Part model, mm, in its own coordinate system. A direction names the side the tool comes from. Coordinates: 2 decimals unless noted, no trailing zeros. Loops run counter-clockwise (first coordinate to the right, second up) from the corner with the lowest first, then second, coordinate; pieces in that order, holes last. Notation, with made-up numbers: (77, 5.25) - (100, 5.25) arc R17 cw to (100, 13.25) - close; hole circle Ø10 at (89, 60.25). An arc over 180 degrees is marked (long way). Use a Markdown table: item, result. Add a question column.
1. Drop flat-ended pins along their axis: pin 1 (2 mm diameter, centred on x = 1, z = 5.5, fed in from -Y); pin 2 (0.5 mm diameter, centred on y = 1, z = 0, fed in from +X); pin 3 (2 mm diameter, centred on x = 1, z = 7, fed in from +Y). Give the stop position or say it passes through.
2. Band-saw the part on A-A, the plane z = 5. Give the cut face in (x, y), plus the area to 3 significant figures.
3. Pull direction Y, two halves, no side cores. Call faces 3 (the flat face through (0.7, 0.6, 0)), 4 (the conical face through (0.35, -0.05, 1.22)), 5 (the cylindrical face through (-2.23, -0.29, 1.35)): pulls with the +Y half, pulls with the -Y half, needs draft (parallel to the pull), parting line crosses it, or undercut.
4. 3-axis set-ups, long thin cutter, end or side, ignore diameter. For faces 1 (the cylindrical face through (-1.29, -0.17, 11.84)), 2 (the flat face through (-0.7, 0.6, 0)): which of +Z, -Z, +X, -X, +Y, -Y reach the whole face in a straight line?
5. Wall check: probe 1 along X at (y, z) = (-0.05, 6.75); probe 2 along Z at (x, y) = (-1.1, -1.15); probe 3 along X at (y, z) = (-0.45, 13.75). Give the ranges that are in metal, low to high. Write a range as [from, to].
Autodesk Inventor part; units mm, degrees
ref_plane "YZ Plane" through (0, 0, 0) normal (1, 0, 0) x (0, 1, 0)
ref_plane "XZ Plane" through (0, 0, 0) normal (0, 1, 0) x (-1, 0, 0)
ref_plane "XY Plane" through (0, 0, 0) normal (0, 0, 1) x (1, 0, 0)
sketch "スケッチ1" plane through (0, 0, 0) normal (1, 0, 0) x (0, 1, 0)
  line L0 (0, 21.7) -> (0, 0)
  line L1 (0, 0) -> (1.25, 0)
  line L2 (2.25, 1) -> (2.25, 1.7)
  line L3 (2.25, 1.7) -> (1.3, 1.7)
  line L4 (1.3, 1.7) -> (1.3, 21.7)
  line L5 (1.3, 21.7) -> (0, 21.7)
  line L6 (1.25, 0) -> (0, 1.7)
  arc A0 (1.25, 0) -> (2.25, 1) centre (1.25, 1) ccw
  line L7 (1.25, 0) -> (2.25, 0)
  line L8 (2.25, 0) -> (2.25, 1)
  dimension "d2" = 1.7
  dimension "d10" = 20
  dimension "d11" = 2.6
  dimension "d12" = 4.5
  dimension "d14" = 1
revolve "回転1" add sketch "スケッチ1" angle 360 about axis through (0, 0, 21.7) along (0, 0, -1) contours L5 L4 L3 L2 A0 L6 L0
thread "ねじ1"
sketch "スケッチ2" plane through (0, 0, 1.7) normal (0, 0, 1) x (1, 0, 0)
  line L0 (0.3339, -1.6357) -> (-0.3339, -1.6357)
  line L1 (-0.3339, -1.6357) -> (-0.3339, -0.7226)
  line L2 (-0.3339, 1.6357) -> (0.3339, 1.6357)
  line L3 (0.3339, 1.6357) -> (0.3339, 0.7226)
  line L4 (0.3339, -1.6357) -> (-0.3339, 1.6357) construction
  line L5 (-0.3339, -1.6357) -> (0.3339, 1.6357) construction
  line L6 (-1.5922, 0.2226) -> (-0.8339, 0.2226)
  line L7 (1.5922, 0.2226) -> (1.5922, -0.2226)
  line L8 (1.5922, -0.2226) -> (0.8339, -0.2226)
  line L9 (-1.5922, -0.2226) -> (-1.5922, 0.2226)
  line L10 (-1.5922, 0.2226) -> (1.5922, -0.2226) construction
  line L11 (1.5922, 0.2226) -> (-1.5922, -0.2226) construction
  circle A0 centre (0, 0) radius 2.25
  line L12 (0.3339, -0.7226) -> (0.3339, -1.6357)
  line L13 (0.8339, 0.2226) -> (1.5922, 0.2226)
  line L14 (-0.8339, -0.2226) -> (-1.5922, -0.2226)
  line L15 (-0.3339, 0.7226) -> (-0.3339, 1.6357)
  arc A1 (0.8339, -0.2226) -> (0.3339, -0.7226) centre (0.8339, -0.7226) ccw
  arc A2 (0.3339, 0.7226) -> (0.8339, 0.2226) centre (0.8339, 0.7226) ccw
  arc A3 (-0.8339, 0.2226) -> (-0.3339, 0.7226) centre (-0.8339, 0.7226) ccw
  arc A4 (-0.3339, -0.7226) -> (-0.8339, -0.2226) centre (-0.8339, -0.7226) ccw
  point P0 (0, 0)
  point P1 (-0.3339, -0.2226)
  point P2 (-0.3339, 0.2226)
  point P3 (0.3339, 0.2226)
  point P4 (0.3339, -0.2226)
  dimension "d18" = 0.5
extrude "押し出し2" add sketch "スケッチ2" against normal blind 1.7
revolve "回転2" cut sketch "スケッチ1" angle 360 about axis through (0, 0, 21.7) along (0, 0, -1) contours A0 L8 L7
properties part number "F-2620EB" material "チタン"
Geometry check:
| question | item | result |
|---|---|---|
| 1 | pin 1 | stops at y = -1.3 |
| 1 | pin 2 | stops at x = 1.66 |
| 1 | pin 3 | stops at y = 1.3 |
| 2 | outline | circle Ø2.6 at (0, 0) |
| 2 | area | 5.31 mm^2 |
| 3 | face 3 | needs draft |
| 3 | face 4 | undercut |
| 3 | face 5 | parting line crosses it |
| 4 | face 1 | +Z |
| 4 | face 2 | -Z, +X, -X, +Y, -Y |
| 5 | probe 1 | x = [-1.3, 1.3] |
| 5 | probe 2 | z = [0.06, 1.7] |
| 5 | probe 3 | x = [-1.22, 1.22] |
